The drawing under review shows one solid part. Ordinate dimensions are in mm from its lowest x, y, z. Coordinates: 2 decimals unless noted, no trailing zeros. Write each loop counter-clockwise with the first axis right and the second up, starting at its lowest first coordinate (ties: lowest second). Pieces come first, ordered by that corner, then holes. Notation, with made-up numbers: M 5,48.5 L 20,48.5 A17 cw 20,75.5 Z; hole C 84,-38 d5. An arc over 180 degrees is marked long. Write item = value, one per line.
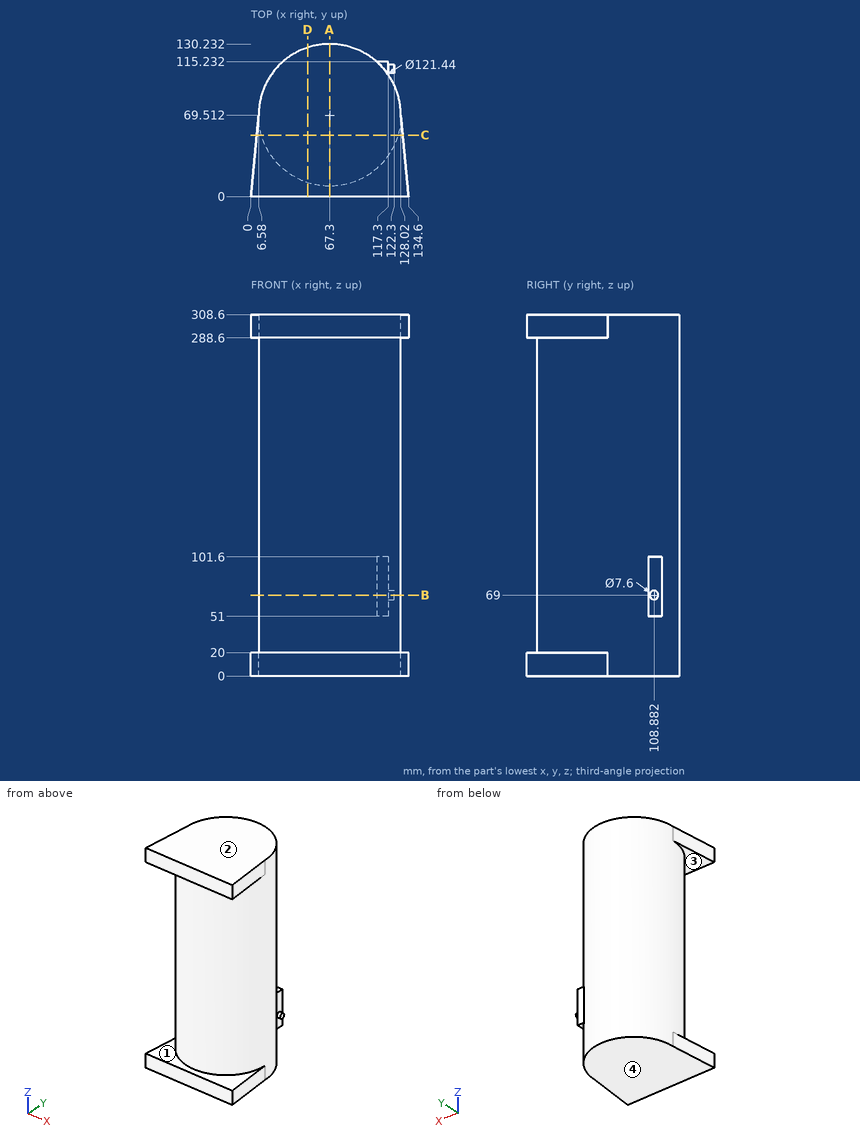
Q1. Consider section C-C, the plane y = 52.5. State the section outline as (x, z) points.
Check result:
outline = M 4.97,0 L 129.63,0 L 129.63,20 L 125.59,20 L 125.59,288.6 L 129.63,288.6 L 129.63,308.6 L 4.97,308.6 L 4.97,288.6 L 9.01,288.6 L 9.01,20 L 4.97,20 Z
Q2. The part is to be moulded in two halves that separate along Z. For the marked faces 1, 2, 3 and 4, say which applies: +Z half, -Z half, draft (parallel to the pull), parting line (faces both ways), or undercut.
Check result:
face_1 = undercut
face_2 = +Z half
face_3 = undercut
face_4 = -Z half
Q3. Consider section D-D, the plane x = 48.5. State the section outline as (y, z) points, and give its area (3 significant figures).
Check result:
outline = M 0,0 L 127.25,0 L 127.25,308.6 L 0,308.6 L 0,288.6 L 11.78,288.6 L 11.78,20 L 0,20 Z
area = 36,100 mm²
Q4. Wall thickness on line 1 (Z direction, x = 110.5, y = 10); line 2 (Y direction, x = 68.5, z = 81.5) (1 decimal); line 3 (Y direction, x = 70, z = 136): over which ranges is each line inside the solid? List them lowest first.
Check result:
line_1 = 0 to 20, 288.6 to 308.6
line_2 = 8.8 to 130.2
line_3 = 8.85 to 130.17
Q5. Consider section A-A, the plane x = 67.3. State the section outline as (y, z) points, and give its area (3 significant figures).
Check result:
outline = M 0,0 L 130.23,0 L 130.23,308.6 L 0,308.6 L 0,288.6 L 8.79,288.6 L 8.79,20 L 0,20 Z
area = 37,800 mm²
Q6. Consider section B-B, the plane z = 69. State the section outline as (x, y) points.
Check result:
outline = M 107.26,115.23 A60.72 ccw long 117.3,103.96 L 117.3,105.08 L 122.3,105.08 L 122.3,112.68 L 117.3,112.68 L 117.3,115.23 Z
Q7. For P1, Ø12.5, axis at y = 112, z = 66, coming from the +X side; P2, Ø4, axis at x = 98.5, z = 50.5, coming from the -Y side (1 decimal); P3, Ø8, axis at x = 113.5, z = 87, coming from the +Y side, all flat-tipped, find the tip position at first contact; note any pin that passes through.
Check result:
P1 = 122.3
P2 = 16.3
P3 = 115.23
